Build history of the part. All positions in model axes, mm. Face numbers are marked on the shaded views. Round coordinates to 2 decimals unless told otherwise and drop trailing zeros. Write each loop counter-clockwise with the first axis right and the second up, starting at its lowest first coordinate (ties: lowest second). Pieces come first, ordered by that corner, then holes. Notation, with made-up numbers: M -6.75,38.5 L 1.25,38.5 A34 cw 1.25,70.5 Z; hole C -39,46 d9. An arc over 180 degrees is marked long. Write item = value, one per line. Start each with the question number.
Q1. Probe L1, parallel to Z at x = -53, y = 107.5; L2, parallel to Y at x = -46, z = -173. List the from-to ranges inside material, lowest first.
Q2. Pull direction Z, two halves, no side cores. Call the marked faces 1, 2 and 3: released by +Z, released by -Z, zero draft, split by the parting line, or undercut.
Q3. Band-saw the part on B-B on x = -28. Write the cut outline in (y, z), plus the area to 3 significant figures.
Q4. Band-saw the part on C-C on z = -290. Write the cut outline in (x, y).
Q5. Band-saw the part on A-A on y = 104. Write the cut outline in (x, z).
Q6. Drop a flat-ended pin along its axis: P1, Ø17.5, axis at x = -31.5, z = -274, coming from the -Y side. Give the stop position or say it passes through.
Solid Edge part; units mm, degrees
sketch "Sketch1" plane through (0, 0, -145.0039) normal (0, 0, 1) x (1, 0, 0)
  line L0 (-22.5, 111.5073) -> (-22.5, 76.5073)
  line L1 (-22.5, 76.5073) -> (-57.5, 76.5073)
  line L2 (-57.5, 76.5073) -> (-57.5, 111.5073)
  line L3 (-57.5, 111.5073) -> (-22.5, 111.5073)
extrude "Protrusion1" add sketch "Sketch1" along normal blind 5
sketch "Sketch2" plane through (-40, 94.0073, -145.0039) normal (0, 0, -1) x (0, 1, 0)
  line L0 (-7.5, -17.5) -> (7.5, -17.5)
  line L1 (7.5, -17.5) -> (7.5, 17.5)
  line L2 (7.5, 17.5) -> (-7.5, 17.5)
  line L3 (-7.5, 17.5) -> (-7.5, -17.5)
extrude "Protrusion2" add sketch "Sketch2" along normal up to vertex (198 mm away)
sketch "Sketch3" plane through (-40, 94.0073, -343.0039) normal (0, 0, -1) x (0, 1, 0)
  line L0 (-17.5, 17.5) -> (-17.5, -17.5)
  line L1 (-17.5, -17.5) -> (17.5, -17.5)
  line L2 (17.5, -17.5) -> (17.5, 17.5)
  line L3 (17.5, 17.5) -> (-17.5, 17.5)
extrude "ExtrudedProtrusion_3" add sketch "Sketch3" along normal blind 5
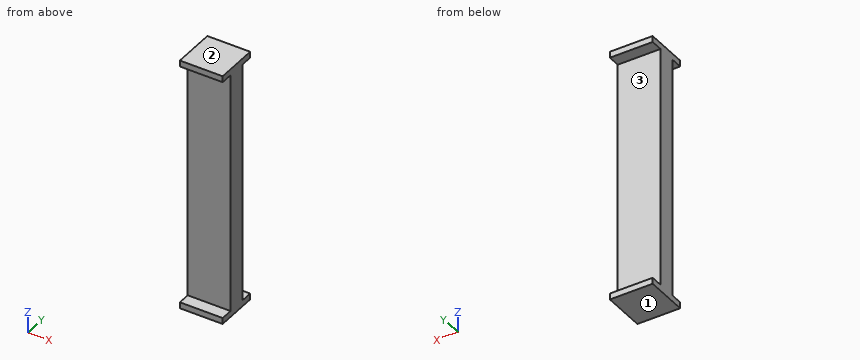
Conclusion:
q1.L1 = -348 to -343, -145 to -140
q1.L2 = 86.51 to 101.51
q2.face_1 = released by -Z
q2.face_2 = released by +Z
q2.face_3 = undercut
q3.outline = M 76.51,-348 L 111.51,-348 L 111.51,-343 L 101.51,-343 L 101.51,-145 L 111.51,-145 L 111.51,-140 L 76.51,-140 L 76.51,-145 L 86.51,-145 L 86.51,-343 L 76.51,-343 Z
q3.area = 3,320 mm^2
q4.outline = M -57.5,86.51 L -22.5,86.51 L -22.5,101.51 L -57.5,101.51 Z
q5.outline = M -57.5,-348 L -22.5,-348 L -22.5,-343 L -57.5,-343 Z; M -57.5,-145 L -22.5,-145 L -22.5,-140 L -57.5,-140 Z
q6.P1 = 86.51
